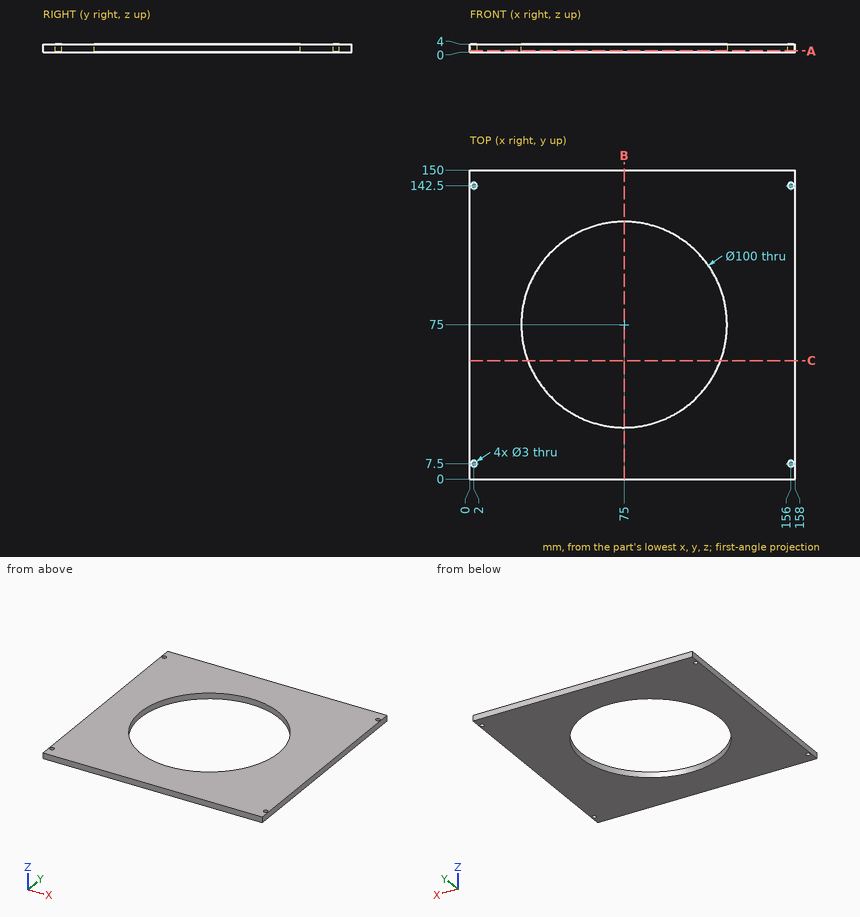
Print and shaded views of the part. All mm, measured from the part's lowest x, y and z. Give positions to 0.01 mm unless a question says otherwise; leave off trailing zeros. Loops run counter-clockwise (first coordinate to the right, second up) from the corner with the lowest first, then second, coordinate; pieces in that order, holes last. Notation, with made-up numbers: (8, 9) -> (51, 9) arc R16 cw to (51, 23) -> close; hole circle Ø8 at (50.5, 15.5). An arc over 180 degrees is marked (long way). Use CSV: the item, a comma, the result in double quotes. Start each with the question number.
1) Slice it at C-C on y = 57.5. Give the cut face in (x, z).
2) Slice it at B-B on x = 75. Give the cut face in (y, z), plus the area to 3 significant figures.
3) Slice it at A-A on z = 0.65. Give the cut face in (x, y), plus the area to 3 significant figures.
4) Flat gauge pin, fed straight in: pin 1 Ø2.5 at (x, y) = (156, 142.5) entering from -Z. Where does the tip first touch, or does it go through?
5) Wall check: line 1 (X direction, y = 142.5, z = 1); line 2 (Y direction, x = 156, z = 2.05); line 3 (Y direction, x = 75, z = 2.75). Give the ranges that are in metal, low to high.
Computed values:
1,outline,"(0, 0) -> (28.16, 0) -> (28.16, 4) -> (0, 4) -> close; (121.84, 0) -> (158, 0) -> (158, 4) -> (121.84, 4) -> close"
2,outline,"(0, 0) -> (25, 0) -> (25, 4) -> (0, 4) -> close; (125, 0) -> (150, 0) -> (150, 4) -> (125, 4) -> close"
2,area,"200 mm^2"
3,outline,"(0, 0) -> (158, 0) -> (158, 150) -> (0, 150) -> close; hole circle Ø3 at (2, 7.5); hole circle Ø3 at (2, 142.5); hole circle Ø100 at (75, 75); hole circle Ø3 at (156, 7.5); hole circle Ø3 at (156, 142.5)"
3,area,"15,800 mm^2"
4,pin 1,"passes through"
5,line 1,"x = 0 to 0.5, 3.5 to 154.5, 157.5 to 158"
5,line 2,"y = 0 to 6, 9 to 141, 144 to 150"
5,line 3,"y = 0 to 25, 125 to 150"
